Input: dimensioned drawing with shaded views. Units: mm. Origin: part minimum x, y, z. A direction names the side the tool comes from. Coordinates: 2 decimals unless noted, no trailing zeros. Loops run counter-clockwise (first coordinate to the right, second up) from the corner with the lowest first, then second, coordinate; pieces in that order, holes last.
(1) Line query: L1, parallel to X at y = 3.5, z = 46; L2, parallel to Y at x = 89, z = 39; L3, parallel to Z at x = 49.5, y = 2.25. Output: solid intervals per line, ascending.
(2) Section D-D, the plane x = 9. Return loops of the section in (y, z), then the cut area to 3 significant figures.
(3) Set-up query: the marked faces 1, 2, 3 and 4. Return all of +Z, -Z, +X, -X, +Y, -Y with unobstructed straight access to the full face (end or side cutting, diameter ignored); none if empty.
(4) Section A-A, the plane y = 3.75. Return loops of the section in (x, z).
(5) Section C-C, the plane x = 68. Return loops of the section in (y, z), then the cut area to 3 significant figures.
(6) Section B-B, the plane z = 54. Return loops of the section in (x, y), then the cut area to 3 significant figures.
(7) Contact query for flat-ended pins moving along their axis: P1, Ø11, axis at x = 86, z = 50, coming from the +Y side; P2, Ø2.5, axis at x = 85, z = 56.5, coming from the -Y side; P3, Ø0.8, axis at x = 26, y = 0.5, coming from the +Z side; P4, Ø6, axis at x = 41.5, z = 45, coming from the -Y side. Output: stop coordinate, or through.
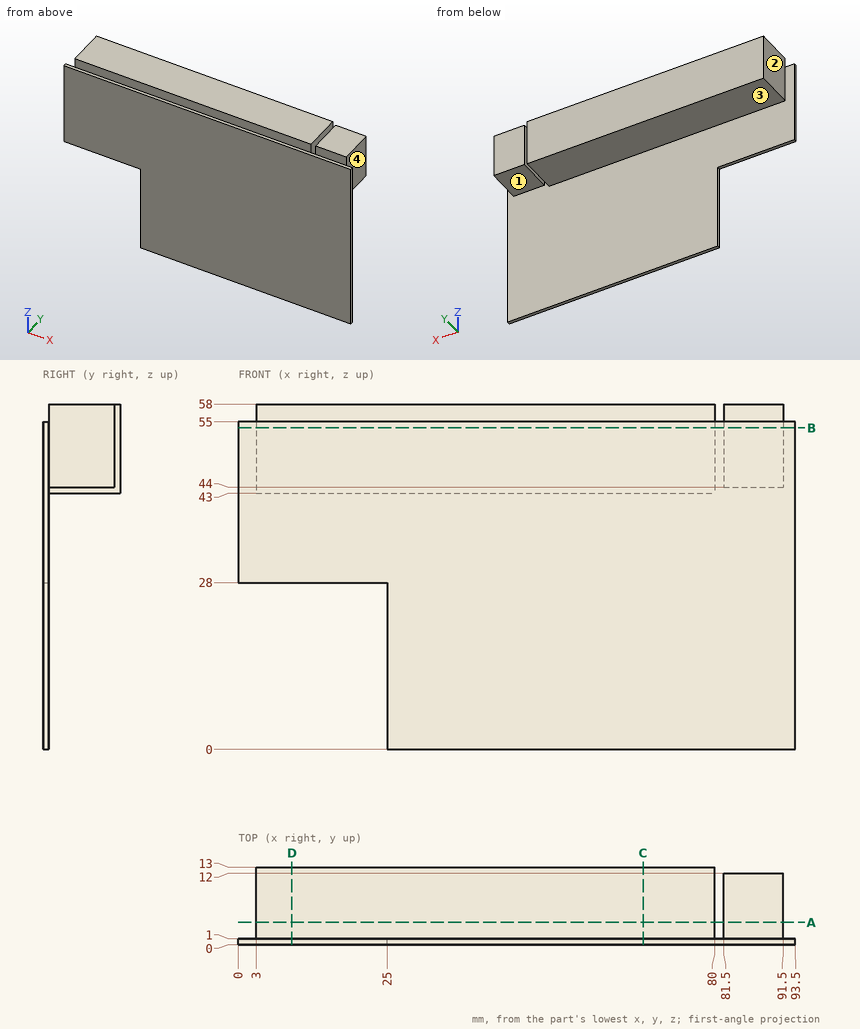
Report:
1. L1: x = 3 to 80, 81.5 to 91.5
1. L2: y = 0 to 1
1. L3: z = 43 to 58
2. outline: (0, 28) - (1, 28) - (1, 43) - (13, 43) - (13, 58) - (1, 58) - (1, 55) - (0, 55) - close
2. area: 207 mm2
3. face 1: -Z, +X, +Y
3. face 2: +Z, -Z, -X, +Y
3. face 3: -Z, +X, -X, +Y
3. face 4: +Z, -Z, +X, +Y
4. outline: (3, 43) - (80, 43) - (80, 58) - (3, 58) - close; (81.5, 44) - (91.5, 44) - (91.5, 58) - (81.5, 58) - close
5. outline: (0, 0) - (1, 0) - (1, 43) - (13, 43) - (13, 58) - (1, 58) - (1, 55) - (0, 55) - close
5. area: 235 mm2
6. outline: (0, 0) - (93.5, 0) - (93.5, 1) - (91.5, 1) - (91.5, 12) - (81.5, 12) - (81.5, 1) - (80, 1) - (80, 13) - (3, 13) - (3, 1) - (0, 1) - close
6. area: 1,130 mm2
7. P1: stops at y = 12
7. P2: stops at y = 1
7. P3: stops at z = 55
7. P4: stops at y = 0
